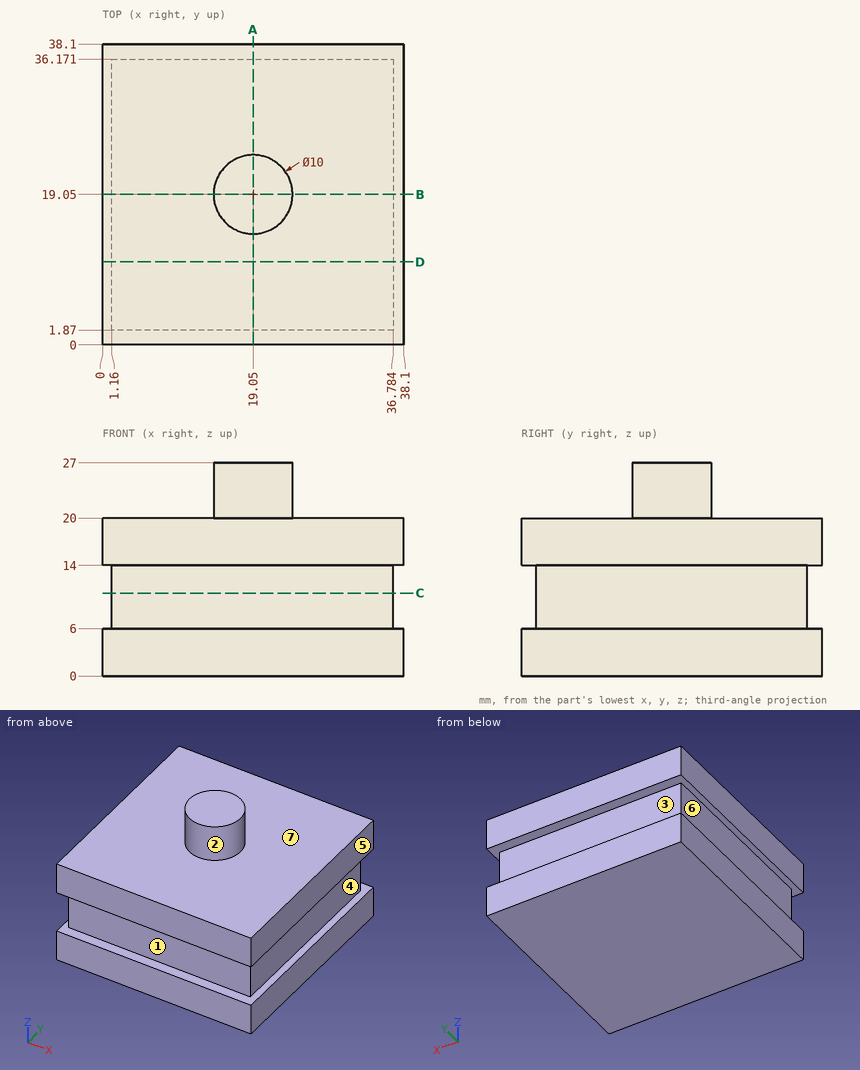
Job drawing, mm, ordinate dimensions from the low corner. One solid piece. A direction names the side the tool comes from. Give positions to 0.01 mm unless a question says otherwise; leave off trailing zeros. Order: outer loops, then holes, each group sorted by start corner. A loop starts at its lowest first (then second) coordinate and runs counter-clockwise, first axis right, second up. Notation, with made-up numbers: (-30.5, -21) - (2.5, -21) arc R20 cw to (2.5, 13) - close; hole circle Ø4 at (67.5, 15). An arc over 180 degrees is marked (long way). Return JSON: item names as keys, results as strings.
1) Cut at D-D, the plane y = 10.5. Give the cut face in (x, z).
Geometry says:
{"outline": "(0, 0) - (38.1, 0) - (38.1, 6) - (36.78, 6) - (36.78, 14) - (38.1, 14) - (38.1, 20) - (0, 20) - (0, 14) - (1.16, 14) - (1.16, 6) - (0, 6) - close"}
2) Cut at C-C, the plane z = 10.5. Give the cut face in (x, y).
Geometry says:
{"outline": "(1.16, 1.87) - (36.78, 1.87) - (36.78, 36.17) - (1.16, 36.17) - close"}
3) Flat gauge pins, fed straight in: P1, Ø5, axis at x = 24.5, y = 5, coming from the +Z side; P2, Ø6.5, axis at y = 25.5, z = 10.5, coming from the -X side; P3, Ø2.5, axis at x = 19, z = 9, coming from the +Y side. Where does each tip first touch, or does it go through?
Geometry says:
{"P1": "z = 20", "P2": "x = 1.16", "P3": "y = 36.17"}
4) Cut at A-A, the plane x = 19.05. Give the cut face in (y, z), plus the area to 3 significant figures.
Geometry says:
{"outline": "(0, 0) - (38.1, 0) - (38.1, 6) - (36.17, 6) - (36.17, 14) - (38.1, 14) - (38.1, 20) - (24.05, 20) - (24.05, 27) - (14.05, 27) - (14.05, 20) - (0, 20) - (0, 14) - (1.87, 14) - (1.87, 6) - (0, 6) - close", "area": "802 mm²"}
5) 3-axis set-ups, long thin cutter, end or side, ignore diameter. For the marked faces 1, 2, 3 and 4: which of +Z, -Z, +X, -X, +Y, -Y reach the whole face in a straight line?
Geometry says:
{"face 1": "+X, -X, -Y", "face 2": "+Z", "face 3": "+X, -X, +Y", "face 4": "+X, +Y, -Y"}
6) Cut at B-B, the plane y = 19.05. Give the cut face in (x, z).
Geometry says:
{"outline": "(0, 0) - (38.1, 0) - (38.1, 6) - (36.78, 6) - (36.78, 14) - (38.1, 14) - (38.1, 20) - (24.05, 20) - (24.05, 27) - (14.05, 27) - (14.05, 20) - (0, 20) - (0, 14) - (1.16, 14) - (1.16, 6) - (0, 6) - close"}
7) Pull direction Z, two halves, no side cores. Call the marked faces 5, 6 and 7: pulls with the +Z half, pulls with the -Z half, needs draft (parallel to the pull), parting line crosses it, or undercut.
Geometry says:
{"face 5": "needs draft", "face 6": "undercut", "face 7": "pulls with the +Z half"}
8) Probe line 1 (Z direction, x = 35, y = 37); line 2 (X direction, y = 21.5, z = 9.25); line 3 (Z direction, x = 7, y = 21). List the from-to ranges inside material, lowest first. Write a range as from..to.
Geometry says:
{"line 1": "0..6, 14..20", "line 2": "1.16..36.78", "line 3": "0..20"}
